```python
from build123d import *
from build123d.topology import SkipClean

# Parameters (mm, degrees)
SKETCH_1_R      = 11
SKETCH_1_R_2    = 2
SKETCH_1_R_3    = 4
EXTRUDE_1_DEPTH = 4
EXTRUDE_START   = 20
SKETCH_2_R      = 5.5
SKETCH_2_R_2    = 4
EXTRUDE_2_DEPTH = 20
EXTRUDE_START_2 = 3
SKETCH_3_R      = 7
SKETCH_3_R_2    = 4
EXTRUDE_3_DEPTH = 3


with BuildPart() as part:
    # 草图1 → 凸台-拉伸1 (new body)
    with BuildSketch(Plane.XY):
        Circle(SKETCH_1_R)
        with Locations((0, 8)):
            Circle(SKETCH_1_R_2, mode=Mode.SUBTRACT)
        with Locations((8, 0)):
            Circle(SKETCH_1_R_2, mode=Mode.SUBTRACT)
        with Locations((0, -8)):
            Circle(SKETCH_1_R_2, mode=Mode.SUBTRACT)
        with Locations((-8, 0)):
            Circle(SKETCH_1_R_2, mode=Mode.SUBTRACT)
        Circle(SKETCH_1_R_3, mode=Mode.SUBTRACT)
    extrude(amount=EXTRUDE_1_DEPTH)

    # 草图2 → 凸台-拉伸2 (add)
    with SkipClean():  # the faces are left unmerged after this step: merging them gives an invalid solid
        with BuildSketch(Plane(origin=(0, 0, 0), x_dir=(-1, 0, 0), z_dir=(0, 0, -1)).offset(EXTRUDE_START)):
            with Locations(Location((0, 0, 0), (0, 0, 180))):
                Circle(SKETCH_2_R)
            Circle(SKETCH_2_R_2, mode=Mode.SUBTRACT)
        extrude(amount=-EXTRUDE_2_DEPTH)

    # 草图3 → 凸台-拉伸3 (add)
    with SkipClean():  # the faces are left unmerged after this step: merging them gives an invalid solid
        with BuildSketch(Plane(origin=(0, 0, -20), x_dir=(-1, 0, 0), z_dir=(0, 0, -1)).offset(EXTRUDE_START_2)):
            Circle(SKETCH_3_R)
            Circle(SKETCH_3_R_2, mode=Mode.SUBTRACT)
        extrude(amount=-EXTRUDE_3_DEPTH)


solid = part.part
```
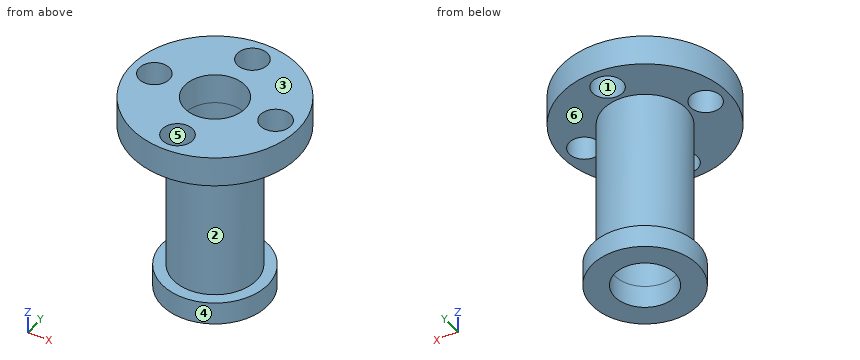
Geometry: final body of the model. Coordinates: model frame, mm. Face numbers are marked on the shaded views. A direction names the side the tool comes from. Give positions to 0.01 mm unless a question says otherwise; leave off trailing zeros. Write each loop counter-clockwise with the first axis right and the second up, starting at its lowest first coordinate (ties: lowest second). Pieces come first, ordered by that corner, then holes.
1. Line query: probe 1 along Z at (x, y) = (3, 4.75); probe 2 along Y at (x, z) = (-0.25, -6); probe 3 along Z at (x, y) = (-3.25, -6.5). Output: solid intervals per line, ascending.
2. Draft query along Z for the marked faces 1, 2 and 3. Return one class per face: released by +Z, released by -Z, zero draft, split by the parting line, or undercut.
3. Reachability of the marked faces 4, 5 and 6 from +Z, -Z, +X, -X, +Y, -Y: full face, straight path, thin tool, end or side. Return the list, or none.
4. Section query D-D, the plane z = -16.25. Return loops of the section in (x, y), then the cut area to 3 significant figures.
5. Section query C-C, the plane y = 9. Return loops of the section in (x, z), then the cut area to 3 significant figures.
6. Pin query (flat end, axial travel): P1, Ø4, axis at x = 6, y = 7.5, coming from the -Z side; P2, Ø6, axis at x = -6.5, z = -9.5, coming from the -Y side; P3, Ø2, axis at y = 2, z = 0, coming from the -X side. Return the tip coordinate at first contact, or that it passes through.
7. Section query A-A, the plane x = 0. Return loops of the section in (y, z).
Computed:
1. probe 1: z = -23 to -20, 0 to 4
1. probe 2: y = -5.49 to -3.99, 3.99 to 5.49
1. probe 3: z = 0 to 4
2. face 1: zero draft
2. face 2: undercut
2. face 3: released by +Z
3. face 4: -Z
3. face 5: +Z
3. face 6: none
4. outline: circle Ø11 at (0, 0); hole circle Ø8 at (0, 0)
4. area: 44.8 mm2
5. outline: (-6.32, 0) - (-1.73, 0) - (-1.73, 4) - (-6.32, 4) - close; (1.73, 0) - (6.32, 0) - (6.32, 4) - (1.73, 4) - close
5. area: 36.7 mm2
6. P1: stops at z = 0
6. P2: stops at y = -4.24
6. P3: stops at x = -10.95
7. outline: (-11, 0) - (-10, 0) - (-10, 4) - (-11, 4) - close; (-7, -23) - (-4, -23) - (-4, 4) - (-6, 4) - (-6, 0) - (-5.5, 0) - (-5.5, -20) - (-7, -20) - close; (4, -23) - (7, -23) - (7, -20) - (5.5, -20) - (5.5, 0) - (6, 0) - (6, 4) - (4, 4) - close; (10, 0) - (11, 0) - (11, 4) - (10, 4) - close
